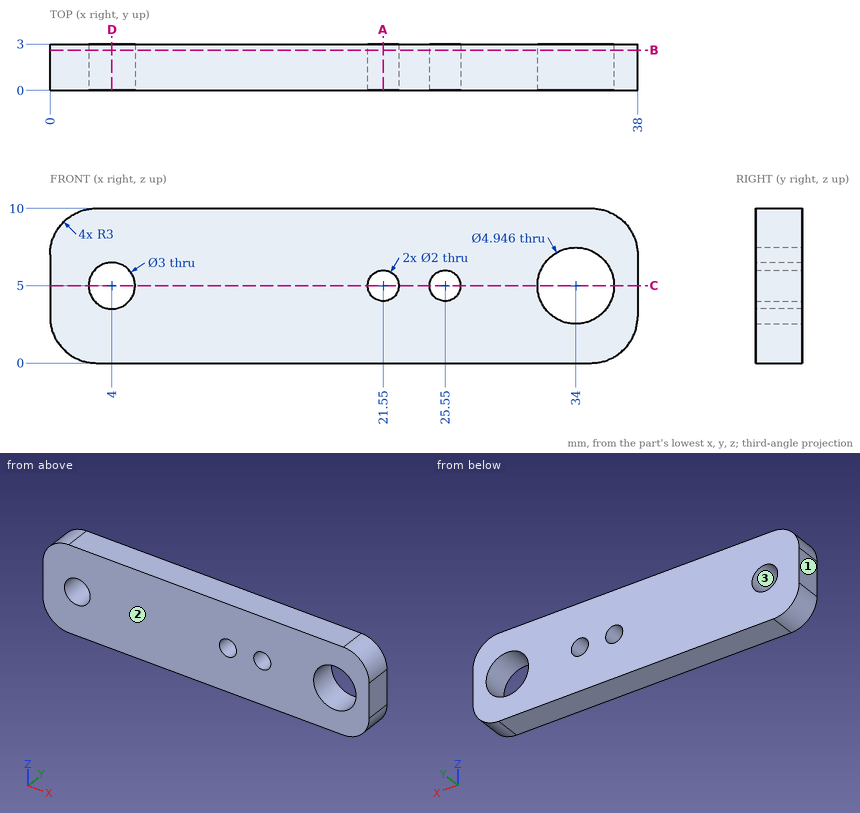
Job drawing, mm, ordinate dimensions from the low corner. One solid piece. Round coordinates to 2 decimals unless told otherwise and drop trailing zeros. Write each loop counter-clockwise with the first axis right and the second up, starting at its lowest first coordinate (ties: lowest second). Pieces come first, ordered by that corner, then holes. Notation, with made-up numbers: M 7.5,18 L 45.5,18 A20 cw 45.5,43 Z; hole C 50.25,25.25 d5. An arc over 180 degrees is marked long. Return JSON: item names as keys, results as strings. Group by question number.
(1) Drill centre lines: probe 1 along X at (y, z) = (0.6, 5); probe 2 along Z at (x, y) = (25.55, 1.75); probe 3 along Z at (x, y) = (4, 1.9). Where is each one in solid material? Low to high.
(2) Saw through at D-D on x = 4. Write the cut outline in (y, z).
(3) Saw through at B-B on y = 2.6. Write the cut outline in (x, z).
(4) Saw through at C-C on z = 5. Write the cut outline in (x, y).
(5) Two-plate mould, pull along X, no slides. Class the marked faces 1, 2 and 3: +X half, -X half, draft (parallel to the pull), parting line (faces both ways), or undercut.
(6) Saw through at A-A on x = 21.55. Write the cut outline in (y, z), then the cut area to 3 significant figures.
(7) Pin check, flat tip, straight feed: pin 1 Ø2.5 at (x, z) = (4, 5) entering from +Y. Stop position of the tip, or through.
Returned:
{
 "1": {"probe 1": "0 to 2.5, 5.5 to 20.55, 22.55 to 24.55, 26.55 to 31.53, 36.47 to 38", "probe 2": "0 to 4, 6 to 10", "probe 3": "0 to 3.5, 6.5 to 10"},
 "2": {"outline": "M 0,0 L 3,0 L 3,3.5 L 0,3.5 Z; M 0,6.5 L 3,6.5 L 3,10 L 0,10 Z"},
 "3": {"outline": "M 0,3 A3 ccw 3,0 L 35,0 A3 ccw 38,3 L 38,7 A3 ccw 35,10 L 3,10 A3 ccw 0,7 Z; hole C 4,5 d3; hole C 21.55,5 d2; hole C 25.55,5 d2; hole C 34,5 d4.95"},
 "4": {"outline": "M 0,0 L 2.5,0 L 2.5,3 L 0,3 Z; M 5.5,0 L 20.55,0 L 20.55,3 L 5.5,3 Z; M 22.55,0 L 24.55,0 L 24.55,3 L 22.55,3 Z; M 26.55,0 L 31.53,0 L 31.53,3 L 26.55,3 Z; M 36.47,0 L 38,0 L 38,3 L 36.47,3 Z"},
 "5": {"face 1": "-X half", "face 2": "draft", "face 3": "undercut"},
 "6": {"outline": "M 0,0 L 3,0 L 3,4 L 0,4 Z; M 0,6 L 3,6 L 3,10 L 0,10 Z", "area": "24.0 mm²"},
 "7": {"pin 1": "through"}
}
